Could you check a few things on this drawing? It's one solid part, dimensions in mm from its lowest x, y, z. Round coordinates to 2 decimals unless told otherwise and drop trailing zeros. Loops run counter-clockwise (first coordinate to the right, second up) from the corner with the lowest first, then second, coordinate; pieces in that order, holes last. Notation, with made-up numbers: (2.25, 42.25) -> (22.25, 42.25) arc R20 cw to (22.25, 71.25) -> close; hole circle Ø7 at (86, 31). An arc over 180 degrees is marked (long way). Write each question's results on one line, items separated by ' | '.
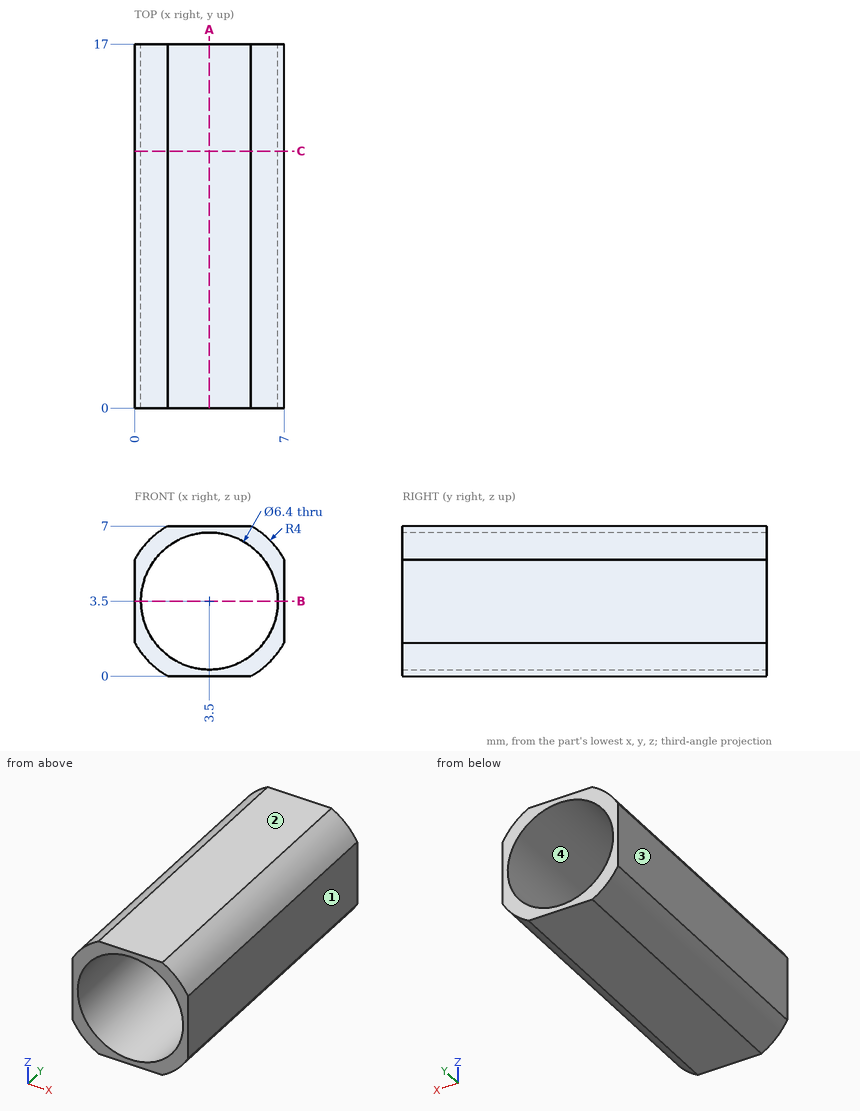
1) I want a section at B-B, the plane z = 3.5. Write out the boundary of the cut face in (x, y), plus the area to 3 significant figures.
Model answer:
outline: (0, 0) -> (0.3, 0) -> (0.3, 17) -> (0, 17) -> close; (6.7, 0) -> (7, 0) -> (7, 17) -> (6.7, 17) -> close | area: 10.2 mm2
2) I need wall thicknesses on line 1 (Z direction, x = 3.5, y = 10); line 2 (X direction, y = 5, z = 5). Which ranges of each line are inside material? Lowest first, please.
Model answer:
line 1: z = 0 to 0.3, 6.7 to 7 | line 2: x = 0 to 0.67, 6.33 to 7
3) I want a section at C-C, the plane y = 12. Write out the boundary of the cut face in (x, z).
Model answer:
outline: (0, 1.56) arc R4 ccw to (1.56, 0) -> (5.44, 0) arc R4 ccw to (7, 1.56) -> (7, 5.44) arc R4 ccw to (5.44, 7) -> (1.56, 7) arc R4 ccw to (0, 5.44) -> close; hole circle Ø6.4 at (3.5, 3.5)
4) If we mould it in two halves opening along X, with no side actions, what happens to the marked faces 1, 2, 3 and 4? For each: released by +X, released by -X, zero draft, split by the parting line, or undercut.
Model answer:
face 1: released by +X | face 2: zero draft | face 3: released by -X | face 4: undercut
5) I want a section at A-A, the plane x = 3.5. Write out the boundary of the cut face in (y, z), plus the area to 3 significant figures.
Model answer:
outline: (0, 0) -> (17, 0) -> (17, 0.3) -> (0, 0.3) -> close; (0, 6.7) -> (17, 6.7) -> (17, 7) -> (0, 7) -> close | area: 10.2 mm2
